Verification items for the finished model (mm, model axes). A direction names the side the tool comes from. Round coordinates to 2 decimals unless told otherwise and drop trailing zeros. Order: outer loops, then holes, each group sorted by start corner. A loop starts at its lowest first (then second) coordinate and runs counter-clockwise, first axis right, second up. Notation, with made-up numbers: (-36.75, -35.75) -> (-18.75, -35.75) arc R14 ccw to (-18.75, -24.75) -> close; hole circle Ø10 at (82, 38.25). An arc over 180 degrees is marked (long way). Put each result on its own line as item: value.
from build123d import *

# Parameters (mm, degrees)
BOSS_EXTRUDE1_DEPTH    = 150
SKETCH2_W              = 40.109469753
SKETCH2_H              = 90
SKETCH2_W_2            = 2
SKETCH2_H_2            = 20
CUT_EXTRUDE1_DEPTH     = 120
SKETCH3_R              = 5
SKETCH3_R_2            = 2
BOSS_EXTRUDE2_DEPTH    = 3
BOSS_EXTRUDE3_START    = -3
SKETCH4_R              = 5
SKETCH4_R_2            = 2
BOSS_EXTRUDE3_DEPTH    = 3
LPATTERN1_COUNT        = 2
LPATTERN1_PITCH        = 120
FILLET1_R              = 60
BOSS_EXTRUDE4_DEPTH    = 1
FILLET2_R              = 20
LPATTERN2_COUNT        = 2
LPATTERN2_PITCH        = 90
FILLET2_OF_LPATTERN2_R = 20
FILLET3_R              = 10


with BuildPart() as part:
    # Sketch1 → Boss-Extrude1 (new body)
    with BuildSketch(Plane.XY):
        with BuildLine():
            ThreePointArc((33.80740392, -9.058666579), (0, -35), (-33.80740392, -9.058666579))
            ThreePointArc((-33.80740392, -9.058666579), (-35.032148792, -8.351559797), (-35.739255573, -9.576304669))
            ThreePointArc((-35.739255573, -9.576304669), (0, -37), (35.739255573, -9.576304669))
            ThreePointArc((35.739255573, -9.576304669), (35.032148792, -8.351559797), (33.80740392, -9.058666579))
        make_face()
    extrude(amount=BOSS_EXTRUDE1_DEPTH)

    # Sketch2 → Cut-Extrude1 (cut)
    with BuildSketch(Plane(origin=(0, 0, 0), x_dir=(1, 0, 0), z_dir=(0, 1, 0))):
        with Locations((-35.054734877, -75)):
            Rectangle(SKETCH2_W, SKETCH2_H)
        with Locations((35.054734877, -75)):
            Rectangle(SKETCH2_W, SKETCH2_H)
        with Locations((32, -15)):
            Rectangle(SKETCH2_W_2, SKETCH2_H_2)
        with Locations((-32, -15)):
            Rectangle(SKETCH2_W_2, SKETCH2_H_2)
        with Locations((-32, -135)):
            Rectangle(SKETCH2_W_2, SKETCH2_H_2)
        with Locations((32, -135)):
            Rectangle(SKETCH2_W_2, SKETCH2_H_2)
    extrude(amount=-CUT_EXTRUDE1_DEPTH, mode=Mode.SUBTRACT)

    # Sketch3 → Boss-Extrude2 (add)
    # profile 1 of 2: a face of its own
    with BuildSketch(Plane(origin=(0, 0, 0), x_dir=(-1, 0, 0), z_dir=(0, 0, -1))):
        with Locations((-38.899671742, -9.317485624)):
            Circle(SKETCH3_R)
        with Locations((-38.899671742, -9.317485624)):
            Circle(SKETCH3_R_2, mode=Mode.SUBTRACT)
    # profile 2 of 2: a face of its own
    with BuildSketch(Plane(origin=(0, 0, 0), x_dir=(-1, 0, 0), z_dir=(0, 0, -1))):
        with Locations((38.899671742, -9.317485624)):
            Circle(SKETCH3_R)
        with Locations(Location((38.899671742, -9.317485624, 0), (0, 0, 180))):
            Circle(SKETCH3_R_2, mode=Mode.SUBTRACT)
    boss_extrude2 = extrude(amount=-BOSS_EXTRUDE2_DEPTH)

    # Sketch4 → Boss-Extrude3 (add)
    # profile 1 of 2: a face of its own
    with BuildSketch(Plane.XY.offset(30).offset(BOSS_EXTRUDE3_START)):
        with Locations((-38.899671742, -9.317485624)):
            Circle(SKETCH4_R)
        with Locations((-38.899671742, -9.317485624)):
            Circle(SKETCH4_R_2, mode=Mode.SUBTRACT)
    # profile 2 of 2: a face of its own
    with BuildSketch(Plane.XY.offset(30).offset(BOSS_EXTRUDE3_START)):
        with Locations((38.899671742, -9.317485624)):
            Circle(SKETCH4_R)
        with Locations(Location((38.899671742, -9.317485624, 0), (0, 0, 180))):
            Circle(SKETCH4_R_2, mode=Mode.SUBTRACT)
    boss_extrude3 = extrude(amount=BOSS_EXTRUDE3_DEPTH)

    # LPattern1: Boss-Extrude2, Boss-Extrude3 ×2
    with Locations(*[(0, 0, i * LPATTERN1_PITCH) for i in range(1, LPATTERN1_COUNT)]):
        add(boss_extrude2)
        add(boss_extrude3)

    # Fillet1
    fillet1_edges = [part.edges().sort_by_distance(p)[0] for p in [
        (34.892782732, -12.308278238, 1.5),
        (-34.892782732, -12.308278238, 1.5),
        (-34.892782732, -12.308278238, 28.5),
        (34.892782732, -12.308278238, 28.5),
        (34.892782732, -12.308278238, 121.5),
        (-34.892782732, -12.308278238, 121.5),
        (-34.892782732, -12.308278238, 148.5),
        (34.892782732, -12.308278238, 148.5),
    ]]
    fillet(fillet1_edges, radius=FILLET1_R)

    # Sketch5 → Boss-Extrude4 (add, symmetric)
    with BuildSketch(Plane(origin=(0, 0, 120), x_dir=(-1, 0, 0), z_dir=(0, 0, -1))):
        with BuildLine():
            Line((15, -35.457721303), (15, -34.166982403))
            Line((15, -34.166982403), (15, -31.622776602))
            ThreePointArc((15, -31.622776602), (0, -35), (-15, -31.622776602))
            Line((-15, -31.622776602), (-15, -33.823069051))
            Line((-15, -33.823069051), (-15, -33.951934532))
            Line((-15, -33.951934532), (-15, -35.457721303))
            ThreePointArc((-15, -35.457721303), (0, -38.5), (15, -35.457721303))
        make_face()
    boss_extrude4 = extrude(amount=BOSS_EXTRUDE4_DEPTH, both=True)

    # Fillet2
    # the kernel refuses this fillet: 20 mm, written as the material it adds along each edge
    with BuildSketch(Plane(origin=(0, 0, 121), x_dir=(0.802187271950027, -0.5970725087636956, 0), z_dir=(0.5970725087636956, 0.802187271950027, 0))) as fillet2_piece_1_section:
        with BuildLine():
            CenterArc((57, -7.599342077), FILLET2_R, 157.668354991, 22.331645009)
            Line((38.5, 0), (38.13, 0.151986842))
            ThreePointArc((38.13, 0.151986842), (37.75, 0.4), (37, 0.4))
            Line((37, 0.4), (36.6, 0))
            Line((36.6, 0), (36.6, -7.599342077))
            Line((36.6, -7.599342077), (37, -7.599342077))
        make_face()
    fillet2_piece_1 = revolve(axis=Axis((0, 0, 121), (0, 0, -1)), revolution_arc=106.67896401, mode=Mode.PRIVATE)
    fillet2_piece_1 = split(fillet2_piece_1, bisect_by=Plane(origin=(-15, -37.318777993, 124.714554063), z_dir=(1, 0, 0)), keep=Keep.TOP, mode=Mode.PRIVATE)
    fillet2_piece_1 = split(fillet2_piece_1, bisect_by=Plane(origin=(15, -37.318777993, 124.714554063), z_dir=(-1, 0, 0)), keep=Keep.TOP, mode=Mode.PRIVATE)
    add(fillet2_piece_1)
    with BuildSketch(Plane(origin=(0, 0, 119), x_dir=(0.802187271950027, -0.5970725087636956, 0), z_dir=(0.5970725087636956, 0.802187271950027, 0))) as fillet2_piece_2_section:
        with BuildLine():
            CenterArc((57, 7.599342077), FILLET2_R, 180, 22.331645009)
            Line((37, 7.599342077), (36.6, 7.599342077))
            Line((36.6, 7.599342077), (36.6, 0))
            Line((36.6, 0), (37, -0.4))
            ThreePointArc((37, -0.4), (37.75, -0.4), (38.13, -0.151986842))
            Line((38.13, -0.151986842), (38.5, 0))
        make_face()
    fillet2_piece_2 = revolve(axis=Axis((0, 0, 119), (0, 0, -1)), revolution_arc=106.67896401, mode=Mode.PRIVATE)
    fillet2_piece_2 = split(fillet2_piece_2, bisect_by=Plane(origin=(-15, -37.318777993, 115.285445937), z_dir=(1, 0, 0)), keep=Keep.TOP, mode=Mode.PRIVATE)
    fillet2_piece_2 = split(fillet2_piece_2, bisect_by=Plane(origin=(15, -37.318777993, 115.285445937), z_dir=(-1, 0, 0)), keep=Keep.TOP, mode=Mode.PRIVATE)
    add(fillet2_piece_2)

    # LPattern2: Boss-Extrude4 ×2
    with Locations(*[(0, 0, -i * LPATTERN2_PITCH) for i in range(1, LPATTERN2_COUNT)]):
        add(boss_extrude4)

    # Fillet2 of LPattern2
    # the kernel refuses this fillet: 20 mm, written as the material it adds along each edge
    with BuildSketch(Plane(origin=(0, 0, 31), x_dir=(0.802187271950026, -0.597072508763697, 0), z_dir=(0.597072508763697, 0.802187271950026, 0))) as fillet2_of_lpattern2_piece_1_section:
        with BuildLine():
            CenterArc((57, -7.599342077), FILLET2_OF_LPATTERN2_R, 157.668354991, 22.331645009)
            Line((38.5, 0), (38.13, 0.151986842))
            ThreePointArc((38.13, 0.151986842), (37.75, 0.4), (37, 0.4))
            Line((37, 0.4), (36.6, 0))
            Line((36.6, 0), (36.6, -7.599342077))
            Line((36.6, -7.599342077), (37, -7.599342077))
        make_face()
    fillet2_of_lpattern2_piece_1 = revolve(axis=Axis((0, 0, 31), (0, 0, -1)), revolution_arc=106.67896401, mode=Mode.PRIVATE)
    fillet2_of_lpattern2_piece_1 = split(fillet2_of_lpattern2_piece_1, bisect_by=Plane(origin=(15, -37.318777993, 34.714554063), z_dir=(-1, 0, 0)), keep=Keep.TOP, mode=Mode.PRIVATE)
    fillet2_of_lpattern2_piece_1 = split(fillet2_of_lpattern2_piece_1, bisect_by=Plane(origin=(-15, -37.318777993, 34.714554063), z_dir=(1, 0, 0)), keep=Keep.TOP, mode=Mode.PRIVATE)
    add(fillet2_of_lpattern2_piece_1)
    with BuildSketch(Plane(origin=(0, 0, 29), x_dir=(0.8021872719500256, -0.5970725087636976, 0), z_dir=(0.5970725087636976, 0.8021872719500256, 0))) as fillet2_of_lpattern2_piece_2_section:
        with BuildLine():
            CenterArc((57, 7.599342077), FILLET2_OF_LPATTERN2_R, 180, 22.331645009)
            Line((37, 7.599342077), (36.6, 7.599342077))
            Line((36.6, 7.599342077), (36.6, 0))
            Line((36.6, 0), (37, -0.4))
            ThreePointArc((37, -0.4), (37.75, -0.4), (38.13, -0.151986842))
            Line((38.13, -0.151986842), (38.5, 0))
        make_face()
    fillet2_of_lpattern2_piece_2 = revolve(axis=Axis((0, 0, 29), (0, 0, -1)), revolution_arc=106.67896401, mode=Mode.PRIVATE)
    fillet2_of_lpattern2_piece_2 = split(fillet2_of_lpattern2_piece_2, bisect_by=Plane(origin=(-15, -37.318777993, 25.285445937), z_dir=(1, 0, 0)), keep=Keep.TOP, mode=Mode.PRIVATE)
    fillet2_of_lpattern2_piece_2 = split(fillet2_of_lpattern2_piece_2, bisect_by=Plane(origin=(15, -37.318777993, 25.285445937), z_dir=(-1, 0, 0)), keep=Keep.TOP, mode=Mode.PRIVATE)
    add(fillet2_of_lpattern2_piece_2)

    # Fillet3
    # the kernel refuses this fillet: 10 mm, written as the material it adds along each edge
    with BuildSketch(Plane(origin=(15, -6.622776602, 120), x_dir=(1, 0, 0), z_dir=(0, -1, 0))) as fillet3_piece_1_section:
        with BuildLine():
            CenterArc((FILLET3_R, -FILLET3_R), FILLET3_R, 90, 90)
            Line((0, -FILLET3_R), (0, 0))
            Line((0, 0), (FILLET3_R, 0))
        make_face()
    fillet3_piece_1 = extrude(amount=52.200292449, mode=Mode.PRIVATE)
    fillet3_piece_1 = fillet3_piece_1 - Plane(origin=(0, 0, 117.805122466), x_dir=(0.9659258262890681, -0.25881904510252157, 0), z_dir=(0, 0, -1)) * Cylinder(35, 145, mode=Mode.PRIVATE)
    fillet3_piece_1 = fillet3_piece_1 & Plane(origin=(0, 0, 117.805122466), x_dir=(-0.9659258262890681, -0.25881904510252135, 0), z_dir=(0, 0, -1)) * Cylinder(37, 145, mode=Mode.PRIVATE)
    add(fillet3_piece_1)
    with BuildSketch(Plane(origin=(15, -6.622776602, 30), x_dir=(1, 0, 0), z_dir=(0, -1, 0))) as fillet3_piece_2_section:
        with BuildLine():
            CenterArc((FILLET3_R, FILLET3_R), FILLET3_R, 180, 90)
            Line((0, FILLET3_R), (0, 0))
            Line((0, 0), (FILLET3_R, 0))
        make_face()
    fillet3_piece_2 = extrude(amount=52.200292449, mode=Mode.PRIVATE)
    fillet3_piece_2 = fillet3_piece_2 & Plane(origin=(0, 0, 32.194877534), x_dir=(-0.9659258262890681, -0.25881904510252135, 0), z_dir=(0, 0, -1)) * Cylinder(37, 145, mode=Mode.PRIVATE)
    fillet3_piece_2 = fillet3_piece_2 - Plane(origin=(0, 0, 32.194877534), x_dir=(0.9659258262890681, -0.25881904510252157, 0), z_dir=(0, 0, -1)) * Cylinder(35, 145, mode=Mode.PRIVATE)
    add(fillet3_piece_2)
    with BuildSketch(Plane(origin=(-15, -6.622776602, 30), x_dir=(-1, 0, 0), z_dir=(0, -1, 0))) as fillet3_piece_3_section:
        with BuildLine():
            CenterArc((FILLET3_R, -FILLET3_R), FILLET3_R, 90, 90)
            Line((0, -FILLET3_R), (0, 0))
            Line((0, 0), (FILLET3_R, 0))
        make_face()
    fillet3_piece_3 = extrude(amount=52.200292449, mode=Mode.PRIVATE)
    fillet3_piece_3 = fillet3_piece_3 & Plane(origin=(0, 0, 32.194882502), x_dir=(-0.9659258262890681, -0.25881904510252135, 0), z_dir=(0, 0, -1)) * Cylinder(37, 145, mode=Mode.PRIVATE)
    fillet3_piece_3 = fillet3_piece_3 - Plane(origin=(0, 0, 32.194882502), x_dir=(0.9659258262890681, -0.25881904510252157, 0), z_dir=(0, 0, -1)) * Cylinder(35, 145, mode=Mode.PRIVATE)
    add(fillet3_piece_3)
    with BuildSketch(Plane(origin=(-15, -6.622776602, 120), x_dir=(-1, 0, 0), z_dir=(0, -1, 0))) as fillet3_piece_4_section:
        with BuildLine():
            CenterArc((FILLET3_R, FILLET3_R), FILLET3_R, 180, 90)
            Line((0, FILLET3_R), (0, 0))
            Line((0, 0), (FILLET3_R, 0))
        make_face()
    fillet3_piece_4 = extrude(amount=52.200292449, mode=Mode.PRIVATE)
    fillet3_piece_4 = fillet3_piece_4 - Plane(origin=(0, 0, 117.805117498), x_dir=(0.9659258262890681, -0.25881904510252157, 0), z_dir=(0, 0, -1)) * Cylinder(35, 145, mode=Mode.PRIVATE)
    fillet3_piece_4 = fillet3_piece_4 & Plane(origin=(0, 0, 117.805117498), x_dir=(-0.9659258262890681, -0.25881904510252135, 0), z_dir=(0, 0, -1)) * Cylinder(37, 145, mode=Mode.PRIVATE)
    add(fillet3_piece_4)


solid = part.part
Item 1: Section check D-D on y = -23. State how many separate pieces and enclosed holes the cut face has, then the cut area to 3 significant figures.
Check sheet entries:
separate pieces: 4
enclosed holes: 0
area: 317 mm^2
Item 2: Section check A-A on x = -16.5. Record the boundary of the cut face in (y, z).
Check sheet entries:
outline: (-33.12, 0) -> (-30.87, 0) -> (-30.87, 34.73) -> (-33.12, 34.73) -> close; (-33.12, 115.27) -> (-30.87, 115.27) -> (-30.87, 150) -> (-33.12, 150) -> close
Item 3: Material ranges on L1, parallel to X at y = -11, z = 29; L2, parallel to X at y = -24.5, z = 136 (3 decimals); L3, parallel to X at y = -25.5, z = 129, recorded low to high. Write a range as [from, to].
Check sheet entries:
L1: x = [-43.61, -39.98], [-37.82, -33.23], [33.23, 37.82], [39.98, 43.61]
L2: x = [-27.726, -24.995], [24.995, 27.726]
L3: x = [-26.81, -23.97], [23.97, 26.81]
Item 4: Tool access check on faces 4 (the flat face through (-33, -14, 135)), 5 (the cylindrical face through (-40.49, -10.53, 28.48)). Record the directions out of +Z, -Z, +X, -X, +Y, -Y that give a thin tool (end or side, any length) a straight path to the whole face; none if there is none.
Check sheet entries:
face 4: +Y, -Y
face 5: +Z, -Z
Item 5: Section check B-B on z = 35. Record the boundary of the cut face in (x, y).
Check sheet entries:
outline: (-16.34, -33.2) arc R37 ccw to (-15, -33.82) -> (-15, -34.18) arc R37.33 ccw to (15, -34.18) -> (15, -33.82) arc R37 ccw to (16.34, -33.2) -> (16.34, -30.95) arc R35 cw to (-16.34, -30.95) -> close
Item 6: Section check C-C on x = 19. Record the boundary of the cut face in (y, z).
Check sheet entries:
outline: (-31.75, 0) -> (-29.39, 0) -> (-29.39, 32) -> (-31.75, 32) -> close; (-31.75, 118) -> (-29.39, 118) -> (-29.39, 150) -> (-31.75, 150) -> close
Item 7: Release check for a two-part mould opening along Z. For faces 1 (the cylindrical face through (18.325, -30.519, 32.554)), 2 (the cylindrical face through (41.743, -5.205, 148.479)), 3 (the flat face through (38, -12, 147)) record: +Z half, -Z half, draft (parallel to the pull), parting line (faces both ways), or undercut.
Check sheet entries:
face 1: undercut
face 2: draft
face 3: undercut
Item 8: Gauge pin test, flat ends, axial feed: pin 1 Ø5.5 at (y, z) = (-13.5, 133) entering from +X; pin 2 Ø5 at (x, z) = (13.5, 117) entering from -Y; pin 3 Ø2 at (y, z) = (-18, 132.5) entering from -X. Record the tip position at first contact, or that the pin passes through.
Check sheet entries:
pin 1: stops at x = 35.4
pin 2: stops at y = -36.58
pin 3: stops at x = -31
